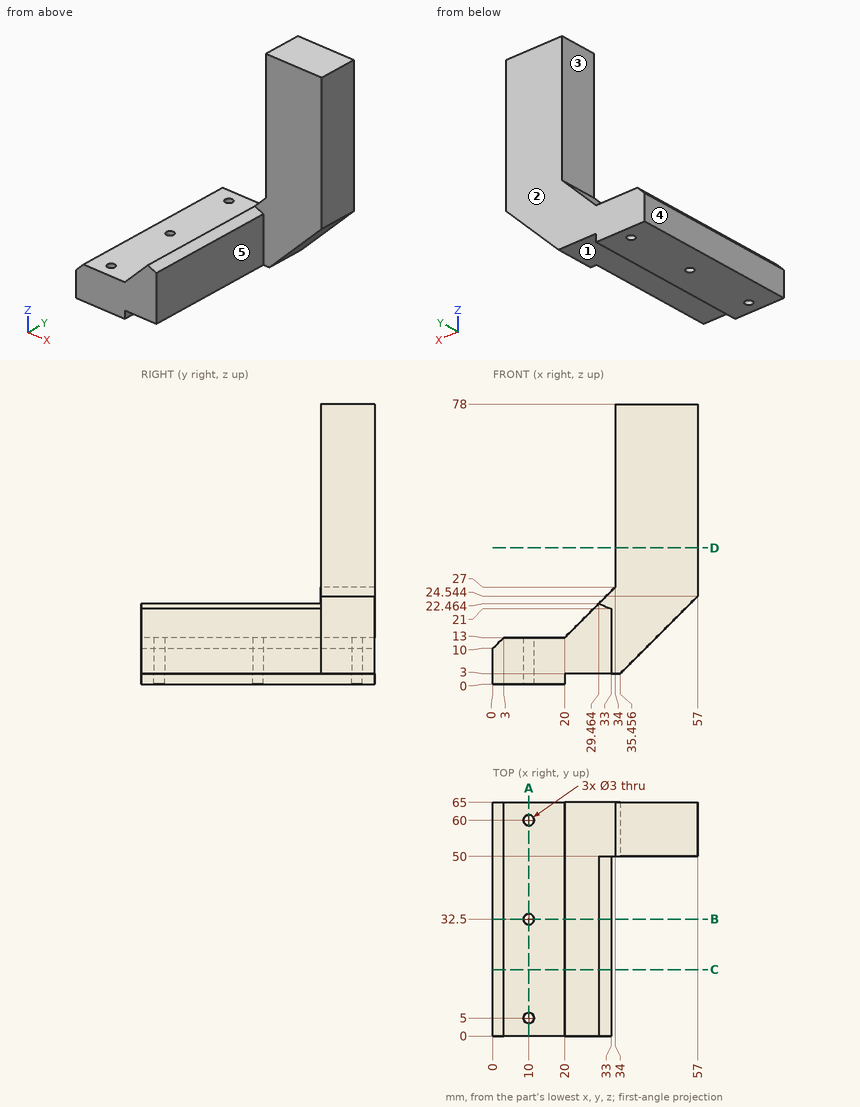
Input: dimensioned drawing with shaded views. Units: mm. Origin: part minimum x, y, z. A direction names the side the tool comes from. Coordinates: 2 decimals unless noted, no trailing zeros. Loops run counter-clockwise (first coordinate to the right, second up) from the corner with the lowest first, then second, coordinate; pieces in that order, holes last. Notation, with made-up numbers: M -12.75,-30 L 3.25,-30 A32 ccw 3.25,-2 Z; hole C 13,87 d2. An arc over 180 degrees is marked long. Use a Markdown table: item, result. Add a question column.
Q1. Material intervals for L1, parallel to Y at x = 10, z = 0.85; L2, parallel to X at y = 32.5, z = 7.5; L3, parallel to X at y = 5, z = 1, sorted ascending.
Q2. Section query B-B, the plane y = 32.5. Return loops of the section in (x, z) (1 decimal), and give its area (3 significant figures).
Q3. Section query A-A, the plane x = 10. Return loops of the section in (y, z).
Q4. First-contact query: pin 1 (5 mm diameter, centred on x = 10, y = 5, fed in from +Z); pin 2 (1.8 mm diameter, centred on x = 10, y = 32.5, fed in from -Z); pin 3 (12 mm diameter, centred on x = 32.5, y = 53.5, fed in from -Z); pin 4 (20 mm diameter, centred on y = 34, z = 14.5, fed in from +X). Flat tips, straight axial feed; report the tip coordinate or a pass-through.
Q5. Section query D-D, the plane z = 38. Return loops of the section in (x, y), and give its area (3 significant figures).
Q6. Section query C-C, the plane y = 18.5. Return loops of the section in (x, z) (1 decimal), and give its area (3 significant figures).
Q7. Access query for the marked faces 1, 2, 3, 4 and 5. Directions: +Z, -Z, +X, -X, +Y, -Y. A direction counts if a zero-diameter tool reaches every point of the face in a straight line with its end or side. Return the directions, or none.
Result:
| question | item | result |
|---|---|---|
| 1 | L1 | y = 0 to 3.5, 6.5 to 31, 34 to 58.5, 61.5 to 65 |
| 1 | L2 | x = 0 to 8.5, 11.5 to 33 |
| 1 | L3 | x = 0 to 8.5, 11.5 to 20 |
| 2 | outline | M 0,0 L 8.5,0 L 8.5,13 L 3,13 L 0,10 Z; M 11.5,0 L 20,0 L 20,3 L 33,3 L 33,21 L 29.5,22.5 L 20,13 L 11.5,13 Z |
| 2 | area | 422 mm2 |
| 3 | outline | M 0,0 L 3.5,0 L 3.5,13 L 0,13 Z; M 6.5,0 L 31,0 L 31,13 L 6.5,13 Z; M 34,0 L 58.5,0 L 58.5,13 L 34,13 Z; M 61.5,0 L 65,0 L 65,13 L 61.5,13 Z |
| 4 | pin 1 | stops at z = 13 |
| 4 | pin 2 | passes through |
| 4 | pin 3 | stops at z = 3 |
| 4 | pin 4 | stops at x = 33 |
| 5 | outline | M 34,50 L 57,50 L 57,65 L 34,65 Z |
| 5 | area | 345 mm2 |
| 6 | outline | M 0,0 L 20,0 L 20,3 L 33,3 L 33,21 L 29.5,22.5 L 20,13 L 3,13 L 0,10 Z |
| 6 | area | 461 mm2 |
| 7 | face 1 | -Z, +X, +Y, -Y |
| 7 | face 2 | +Z, -Z, +X, -X, +Y |
| 7 | face 3 | +Z, -X, +Y, -Y |
| 7 | face 4 | +Z, -Z, -X, +Y, -Y |
| 7 | face 5 | +Z, -Z, +X, -Y |
